from build123d import *

# Parameters (mm, degrees)
EXTRUDE_1_DEPTH = 50
CHAMFER_1_SIZE  = 0.2


with BuildPart() as part:
    # 草圖1 → 填料-伸長1 (new body)
    with BuildSketch(Plane.XY.offset(52)):
        with BuildLine():
            Line((1.984313483, 2.25), (-1.984313483, 2.25))
            ThreePointArc((-1.984313483, 2.25), (0, -3), (1.984313483, 2.25))
        make_face()
    extrude(amount=-EXTRUDE_1_DEPTH)

    # 導角1
    chamfer_1_edges = [part.edges().sort_by_distance(p)[0] for p in [
        (0, 2.25, 52),
        (0, -3, 52),
        (0, -3, 2),
        (0, 2.25, 2),
    ]]
    chamfer(chamfer_1_edges, length=CHAMFER_1_SIZE)


solid = part.part
The listing builds one solid part. Answer for the finished solid, in the listing's coordinates (mm). Coordinates: 2 decimals unless noted, no trailing zeros. Write each loop counter-clockwise with the first axis right and the second up, starting at its lowest first coordinate (ties: lowest second). Pieces come first, ordered by that corner, then holes. Notation, with made-up numbers: (44.5, 15) - (101.5, 15) arc R21 ccw to (101.5, 42) - close; hole circle Ø7 at (55.25, 5.25). An arc over 180 degrees is marked (long way). Answer as CSV lines item,"result".
1. Find section A-A (z = 43). Give the vertices of the cut face in (x, y), plus the area to 3 significant figures.
Computed values:
outline,"(-1.98, 2.25) arc R3 ccw (long way) to (1.98, 2.25) - close"
area,"26.2 mm²"
2. Given P1, Ø1.5, axis at y = -1, z = 27.5, coming from the +X side, flat-ended and moving along its own axis, determine where the tip first touches the part or whether it passes through.
Computed values:
P1,"stops at x = 2.99"
3. Straight lines are drawn through the part: line 1 (X direction, y = -0.25, z = 18); line 2 (Y direction, x = 1.1, z = 5.5); line 3 (Y direction, x = -0.4, z = 6). For each, find the intervals that lie inside material, in ascending order. Write a range as [from, to].
Computed values:
line 1,"x = [-2.99, 2.99]"
line 2,"y = [-2.79, 2.25]"
line 3,"y = [-2.97, 2.25]"
